Could you check a few things on this model? Use its own coordinates, in mm. A direction names the side the tool comes from. Coordinates: 2 decimals unless noted, no trailing zeros. Write each loop counter-clockwise with the first axis right and the second up, starting at its lowest first coordinate (ties: lowest second). Pieces come first, ordered by that corner, then holes.
Item 1: I want a section at A-A on x = 0. Please give me the cut outline in (y, z), then the cut area to 3 significant figures.
Item 2: I want a section at D-D on z = 1.5. Please give me the cut outline in (x, y).
Item 3: I want a section at C-C on z = 20.5. Please give me the cut outline in (x, y).
Item 4: If I drill on probe 1 along Y at (x, z) = (0, 18); probe 2 along Z at (x, y) = (-11.5, 13.5); probe 3 along Z at (x, y) = (1.5, 3), over which ranges is the centre line in solid material (lowest first)?
Item 5: For P1, Ø8, axis at x = 6.5, y = -12.5, coming from the +Z side; P2, Ø1.5, axis at x = 10.5, z = 3, coming from the +Y side; P3, Ø2, axis at x = -15, y = 14, coming from the -Z side, each with a flat end and sliding along its axis, tell me the tip position at first contact or that it passes through.
Item 6: Thinking about a two-plate mould opening in Y: for faces 1 (the flat face through (2, -2, 25)), 2 (the cylindrical face through (-0.338, -2.578, 14.353)), 3 (the flat face through (0, 0, 4)), 4 (the cylindrical face through (-8.46, 6.182, -3.451)), which applies, +Y half, -Y half, draft (parallel to the pull), parting line (faces both ways), or undercut?
Item 7: Which directions (+Z, -Z, +X, -X, +Y, -Y) give clear straight access to the entire face, cutting with the end or side of a thin tool? Please do faces 5 (the cylindrical face through (-4.336, 19.524, 1.972)), 6 (the flat face through (4, -4, 4)).
Autodesk Fusion 360 part; units mm, degrees
sketch "Boceto1" plane through (0, 0, 0) normal (0, 0, 1) x (1, 0, 0)
  circle A0 centre (0, 0) radius 20
  circle A1 centre (0, 0) radius 2.6
  circle A2 centre (-7.8095, 9.1111) radius 3
  dimension "d1" = 40
  dimension "d2" = 5.2
  dimension "d20" = 6
  dimension "d21" = 12
extrude "Extruir1" add sketch "Boceto1" along normal blind 4 contours A0 | A1 | A2
sketch "Boceto2" plane through (0, 0, 4) normal (0, 0, 1) x (1, 0, 0)
  circle A0 centre (0, 0) radius 20
  circle A1 centre (0, 0) radius 2.6
  circle A2 centre (0, 0) radius 5
  dimension "d14" = 5.2
  dimension "d15" = 10
extrude "Extruir2" add sketch "Boceto2" along normal blind 21 contours A2
sketch "Boceto3" plane through (0, 0, 0) normal (1, 0, 0) x (0, 0, -1)
  circle A0 centre (-22, 0) radius 1
  dimension "d18" = 2
extrude "Extruir4" add sketch "Boceto1" against normal blind 8 contours A2
fillet "Empalme1" radius 1 1 edges at (-10.6065, 10.1959, -8)
Response values:
1. outline: (-20, 0) - (20, 0) - (20, 4) - (5, 4) - (5, 25) - (2.6, 25) - (2.6, 4) - (-2.6, 4) - (-2.6, 25) - (-5, 25) - (-5, 4) - (-20, 4) - close
1. area: 261 mm2
2. outline: circle Ø40 at (0, 0)
3. outline: circle Ø10 at (0, 0); hole circle Ø5.2 at (0, 0)
4. probe 1: y = -5 to -2.6, 2.6 to 5
4. probe 2: z = 0 to 4
4. probe 3: z = 0 to 25
5. P1: stops at z = 4
5. P2: stops at y = 17.46
5. P3: stops at z = 0
6. face 1: draft
6. face 2: undercut
6. face 3: undercut
6. face 4: parting line
7. face 5: +Z, -Z
7. face 6: +Z
